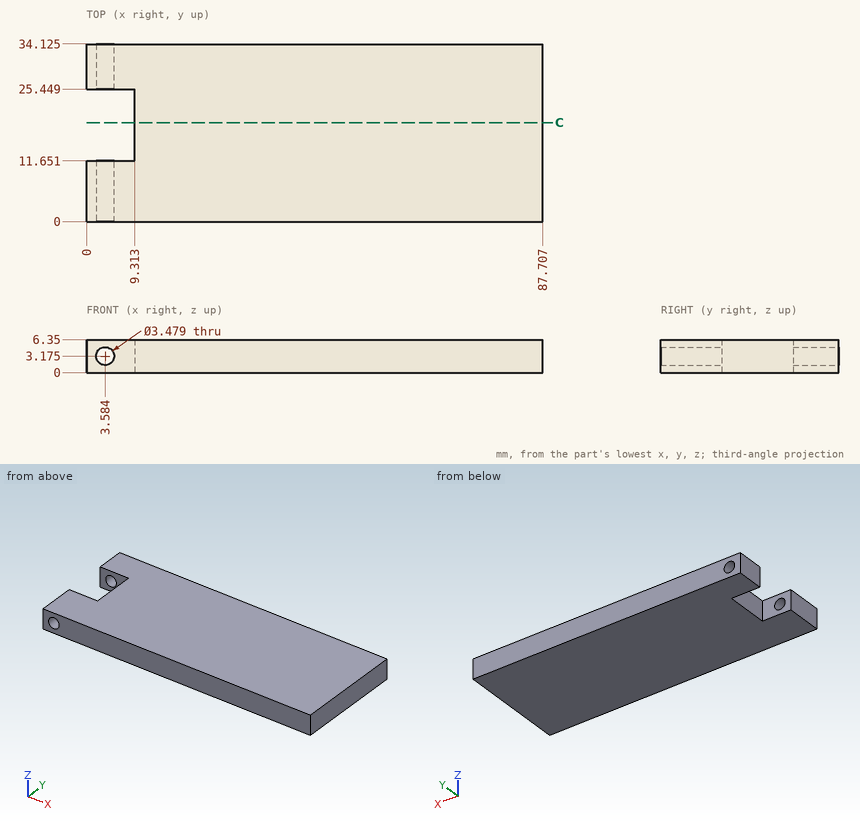
For this review, use the dimensioned drawing (mm, ordinates from the lowest corner) and the shaded views. Give positions to 0.01 mm unless a question says otherwise; leave off trailing zeros. Order: outer loops, then holes, each group sorted by start corner. A loop starts at its lowest first (then second) coordinate and runs counter-clockwise, first axis right, second up. Notation, with made-up numbers: (59.5, 58) - (108.5, 58) arc R12 cw to (108.5, 63) - close; hole circle Ø10 at (74.25, 68). An arc over 180 degrees is marked (long way). Use CSV: the item, a comma, the result in double quotes. Start each with the question number.
Q1. For line 1 (X direction, y = 14.5, z = 4.5); line 2 (X direction, y = 7, z = 2.75); line 3 (X direction, y = 11.5, z = 3.75) (1 decimal), list the stretches that pass through material, from the lowest coordinate up.
Q2. Take a section at C-C (y = 19). State the section outline as (x, z) points, and give its area (3 significant figures).
Q3. For P1, Ø1.9, axis at y = 21, z = 4, coming from the -X side, flat-tipped, find the tip position at first contact; note if it passes through.
Calculated:
1,line 1,"x = 9.31 to 87.71"
1,line 2,"x = 0 to 1.9, 5.27 to 87.71"
1,line 3,"x = 0 to 1.9, 5.2 to 87.7"
2,outline,"(9.31, 0) - (87.71, 0) - (87.71, 6.35) - (9.31, 6.35) - close"
2,area,"498 mm²"
3,P1,"stops at x = 9.31"
